from build123d import *

# Parameters (mm, degrees)
EXTRUDE1_DEPTH                  = 6.35
SKETCH2_R                       = 63.5
CUT_EXTRUDE1_DEPTH              = 6.35
F_6_32_TAPPED_HOLE1_D           = 2.7051
F_6_32_TAPPED_HOLE1_DEPTH       = 9.398
F_6_32_TAPPED_HOLE1_CBORE_D     = 3.5052
F_6_32_TAPPED_HOLE1_CBORE_DEPTH = 7.112
F_6_32_TAPPED_HOLE1_TIP         = 0.81269403


with BuildPart() as part:
    # Sketch1 → Extrude1 (new body)
    with BuildSketch(Plane(origin=(0, 0, 0), x_dir=(1, 0, 0), z_dir=(0, 1, 0))):
        with BuildLine():
            Line((-69.85, 9.525), (0, 9.525))
            Line((0, 9.525), (0, -9.525))
            Line((0, -9.525), (-69.85, -9.525))
            ThreePointArc((-69.85, -9.525), (-74.340128061, -7.665128061), (-76.2, -3.175))
            Line((-76.2, -3.175), (-76.2, 3.175))
            ThreePointArc((-76.2, 3.175), (-74.340128061, 7.665128061), (-69.85, 9.525))
        make_face()
    extrude(amount=EXTRUDE1_DEPTH)

    # Sketch2 → Cut-Extrude1 (cut)
    with BuildSketch(Plane(origin=(0, 6.35, 0), x_dir=(-1, 0, 0), z_dir=(0, 1, 0))):
        Circle(SKETCH2_R)
    extrude(amount=-CUT_EXTRUDE1_DEPTH, mode=Mode.SUBTRACT)

    # #6-32 Tapped Hole1
    with Locations(Plane(origin=(-69.85, 6.35, 0), x_dir=(0, 0, 1), z_dir=(0, 1, 0))):
        with Locations((0, 0)):
            CounterBoreHole(F_6_32_TAPPED_HOLE1_D / 2, F_6_32_TAPPED_HOLE1_CBORE_D / 2, F_6_32_TAPPED_HOLE1_CBORE_DEPTH, depth=F_6_32_TAPPED_HOLE1_DEPTH)
            with Locations((0, 0, -(F_6_32_TAPPED_HOLE1_DEPTH + F_6_32_TAPPED_HOLE1_TIP / 2))):  # 118° drill point
                Cone(0, F_6_32_TAPPED_HOLE1_D / 2, F_6_32_TAPPED_HOLE1_TIP, mode=Mode.SUBTRACT)


solid = part.part
For this review, take the finished solid that the model builds, in its own axes (mm). Coordinates: 2 decimals unless noted, no trailing zeros. Write each loop counter-clockwise with the first axis right and the second up, starting at its lowest first coordinate (ties: lowest second). Pieces come first, ordered by that corner, then holes. Notation, with made-up numbers: (-33, 52) -> (-24, 52) arc R20 ccw to (-24, 86) -> close; hole circle Ø10 at (19.25, -35.5). An arc over 180 degrees is marked (long way). Write each question's results on one line, items separated by ' | '. Start each with the question number.
1) Consider section A-A (z = 0). Write out the cut boundary in (x, y), plus the area to 3 significant figures.
2) The part is to be moulded in two halves that separate along Z. For faces 1 (the face through (-74.29, 3.131, 7.714)), 2 (the face through (-67.9, 0, -0.1)), 3 (the face through (-71.56, 3.22, -0.38)), say which applies: +Z half, -Z half, draft (parallel to the pull), parting line (faces both ways), or undercut.
3) Consider section B-B (y = 2). Write out the cut boundary in (x, z) (3 decimals).
4) Consider section D-D (z = 7.5). Write out the cut boundary in (x, y), plus the area to 3 significant figures.
5) Insertion check: pin 1 (3 mm diameter, centred on x = -69.85, z = 0, fed in from -Y); pin 2 (3 mm diameter, centred on y = 1.5, z = -2, fed in from +X). Each pin has a flat end and moves straight along its axis. Give the tip position at first contact, or say it passes through.
6) Consider section C-C (x = -69.5). Write out the cut boundary in (y, z) (3 decimals), plus the area to 3 significant figures.
7) Wall thickness on L1, parallel to X at y = 4.5, z = 0; L2, parallel to Z at x = -69.85, y = 5.25 (3 decimals); L3, parallel to Z at x = -68.5, y = 1.25 (3 decimals): over which ranges is each line inside the solid? List them lowest first. Write a range as [from, to].
Geometry says:
1) outline: (-76.2, 0) -> (-71.6, 0) -> (-71.6, 6.35) -> (-76.2, 6.35) -> close; (-68.1, 0) -> (-63.5, 0) -> (-63.5, 6.35) -> (-68.1, 6.35) -> close | area: 58.4 mm^2
2) face 1: +Z half | face 2: draft | face 3: undercut
3) outline: (-76.2, -3.175) arc R6.35 ccw to (-69.85, -9.525) -> (-62.782, -9.525) arc R63.5 cw to (-62.782, 9.525) -> (-69.85, 9.525) arc R6.35 ccw to (-76.2, 3.175) -> close; hole circle Ø3.505 at (-69.85, 0)
4) outline: (-74.5, 0) -> (-63.06, 0) -> (-63.06, 6.35) -> (-74.5, 6.35) -> close | area: 72.7 mm^2
5) pin 1: through | pin 2: x = -63.4
6) outline: (0, -9.525) -> (6.35, -9.525) -> (6.35, -1.717) -> (0, -1.717) -> close; (0, 1.717) -> (6.35, 1.717) -> (6.35, 9.525) -> (0, 9.525) -> close | area: 99.2 mm^2
7) L1: [-76.2, -71.6], [-68.1, -63.5] | L2: [-9.525, -1.753], [1.753, 9.525] | L3: [-9.525, -1.118], [1.118, 9.525]
